Could you check a few things on this model? Use its own coordinates, in mm. A direction names the side the tool comes from. Coordinates: 2 decimals unless noted, no trailing zeros. Loops run counter-clockwise (first coordinate to the right, second up) from the corner with the lowest first, then second, coordinate; pieces in that order, holes last.
1) Thinking about a two-plate mould opening in Z: for faces 3 (the face through (-2, 2, 2)), 4 (the face through (1.7, 4, -3.3)), 5 (the face through (-3.543, 0.986, 8.545)), which applies, released by +Z, released by -Z, zero draft, split by the parting line, or undercut?
2) Imagine slicing it at B-B on x = 0. Please give me the cut outline in (y, z).
3) Will these pins go through, and if not, where does the flat tip stop? P1, Ø2, axis at y = 1, z = -6, coming from the +X side; P2, Ø5.5, axis at x = 0, z = 0, coming from the +Y side; P3, Ø2, axis at x = 2, y = 1.5, coming from the -Z side.
4) Imagine slicing it at A-A on z = 0. Please give me the cut outline in (x, y), plus the area to 3 significant figures.
5) For faces 1 (the face through (2.2, 0, -0.1)), 2 (the face through (3, 3, 1.9)), which set-ups out of +Z, -Z, +X, -X, +Y, -Y let a thin tool reach every point of the face, with its end or its side?
6) If I drill on line 1 along X through (y, z) = (1.8, 0.5); line 2 along Z through (x, y) = (0.25, 1.65); line 3 along Z through (x, y) = (-5.75, 1), over which ranges is the centre line in solid material (lowest first)?
```python
from build123d import *

# Parameters (mm, degrees)
SKETCH1_R           = 9.25
SKETCH1_R_2         = 2.05
BOSS_EXTRUDE1_DEPTH = 4
SKETCH2_R           = 3.55
CUT_EXTRUDE1_DEPTH  = 2
CHAMFER1_SIZE       = 2


with BuildPart() as part:
    # Sketch1 → Boss-Extrude1 (new body)
    with BuildSketch(Plane(origin=(0, 0, 0), x_dir=(1, 0, 0), z_dir=(0, 1, 0))):
        with Locations(Location((0, 0, 0), (0, 0, 270))):
            Circle(SKETCH1_R)
        with Locations(Location((0, 0, 0), (0, 0, 270))):
            Circle(SKETCH1_R_2, mode=Mode.SUBTRACT)
    extrude(amount=BOSS_EXTRUDE1_DEPTH)

    # Sketch2 → Cut-Extrude1 (cut)
    with BuildSketch(Plane(origin=(0, 4, 0), x_dir=(1, 0, 0), z_dir=(0, 1, 0))):
        with Locations(Location((0, 0, 0), (0, 0, 270))):
            Circle(SKETCH2_R)
    extrude(amount=-CUT_EXTRUDE1_DEPTH, mode=Mode.SUBTRACT)

    # Chamfer1
    chamfer1_edges = [part.edges().sort_by_distance(p)[0] for p in [
        (0, 4, -9.25),
    ]]
    chamfer(chamfer1_edges, length=CHAMFER1_SIZE)


solid = part.part
```
Filled in:
1. face 3: undercut
1. face 4: zero draft
1. face 5: split by the parting line
2. outline: (0, -9.25) - (2, -9.25) - (4, -7.25) - (4, -3.55) - (2, -3.55) - (2, -2.05) - (0, -2.05) - close; (0, 2.05) - (2, 2.05) - (2, 3.55) - (4, 3.55) - (4, 7.25) - (2, 9.25) - (0, 9.25) - close
3. P1: stops at x = 7.78
3. P2: stops at y = 2
3. P3: stops at z = -9.2
4. outline: (-9.25, 0) - (-2.05, 0) - (-2.05, 2) - (-3.55, 2) - (-3.55, 4) - (-7.25, 4) - (-9.25, 2) - close; (2.05, 0) - (9.25, 0) - (9.25, 2) - (7.25, 4) - (3.55, 4) - (3.55, 2) - (2.05, 2) - close
4. area: 47.6 mm2
5. face 1: +Z, -Z, +X, -X, -Y
5. face 2: +Y
6. line 1: x = -9.24 to -1.99, 1.99 to 9.24
6. line 2: z = -9.25 to -2.03, 2.03 to 9.25
6. line 3: z = -7.25 to 7.25
